Check sheet for the modelled part. Datum: model origin and axes. Units: mm. Face numbers are marked on the shaded views. A direction names the side the tool comes from. Round coordinates to 2 decimals unless told otherwise and drop trailing zeros. Write each loop counter-clockwise with the first axis right and the second up, starting at its lowest first coordinate (ties: lowest second). Pieces come first, ordered by that corner, then holes.
Item 1: Cross-section at C-C on z = 14.25. Enter the section's corners in (x, y) (3 decimals).
Item 2: Cross-section at B-B on y = 38.1. Enter the section's corners in (x, z) (3 decimals).
Item 3: Release check for a two-part mould opening along Z. For the marked faces 1, 2, 3 and 4 record: +Z half, -Z half, draft (parallel to the pull), parting line (faces both ways), or undercut.
Item 4: Go/stop test with a flat-tipped pin: pin 1 Ø5 at (x, y) = (38.1, 38.1) entering from +Z. Record where the tip stops, or that it passes through.
Item 5: Cross-section at A-A on x = 25.4. Enter the section's corners in (y, z) (3 decimals).
Item 6: Tool access check on the marked faces 5 and 6. Record the directions out of +Z, -Z, +X, -X, +Y, -Y that give a thin tool (end or side, any length) a straight path to the whole face; none if there is none.
Item 7: Cross-section at D-D on x = 12.7. Count the separate pieces of the cut face and the enclosed holes in it, plus the area to 3 significant figures.
Item 8: Material ranges on line 1 (X direction, y = 38.1, z = 23.5) (3 decimals); line 2 (X direction, y = 46, z = 17.75) (3 decimals); line 3 (Z direction, x = 47.5, y = 93.5) (3 decimals), recorded low to high.
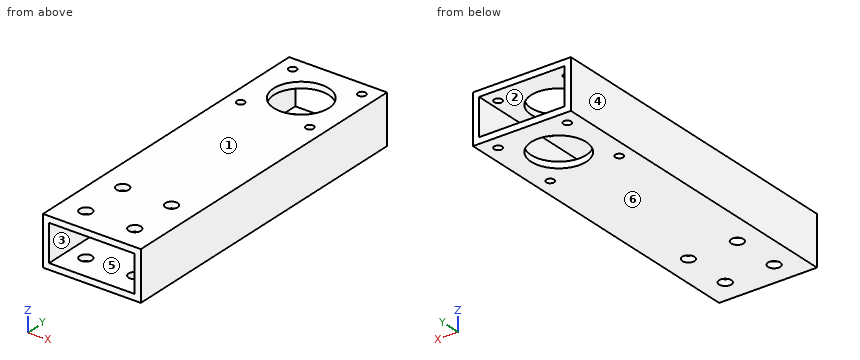
Autodesk Inventor part; units mm, degrees
ref_plane "YZ Plane" through (0, 0, 0) normal (1, 0, 0) x (0, 1, 0)
ref_plane "XZ Plane" through (0, 0, 0) normal (0, 1, 0) x (-1, 0, 0)
ref_plane "XY Plane" through (0, 0, 0) normal (0, 0, 1) x (1, 0, 0)
sketch "Sketch1" plane through (0, 0, 0) normal (0, 0, 1) x (1, 0, 0)
  line L0 (0, 0) -> (50.8, 0)
  line L1 (50.8, 0) -> (50.8, 169.8752)
  line L2 (50.8, 169.8752) -> (0, 169.8752)
  line L3 (0, 169.8752) -> (0, 0)
  line L4 (25.4, 169.8752) -> (25.4, 144.4752)
  line L5 (25.4, 169.8752) -> (50.8, 169.8752) construction
  circle A0 centre (25.4, 144.4752) radius 14.2875
  line L6 (25.4, 144.4752) -> (43.3605, 162.4357)
  line L7 (25.4, 144.4752) -> (50.8, 144.4752) construction
  line L8 (7.4395, 126.5147) -> (43.3605, 126.5147)
  line L9 (43.3605, 162.4357) -> (7.4395, 162.4357)
  line L10 (7.4395, 162.4357) -> (7.4395, 126.5147)
  circle A1 centre (7.4395, 162.4357) radius 2.032
  circle A2 centre (7.4395, 126.5147) radius 2.032
  circle A3 centre (43.3605, 162.4357) radius 2.032
  circle A4 centre (43.3605, 126.5147) radius 2.032
  line L11 (0, 0) -> (50.8, 0)
  line L12 (50.8, 0) -> (50.8, 38.1)
  line L13 (0, 38.1) -> (0, 0)
  line L14 (25.4, 38.1) -> (12.7, 38.1)
  line L15 (25.4, 38.1) -> (38.1, 38.1) construction
  line L16 (12.7, 38.1) -> (38.1, 38.1)
  circle A5 centre (12.7, 38.1) radius 3.175
  circle A6 centre (38.1, 38.1) radius 3.175
  dimension "d0" = 50.8
  dimension "d1" = 169.8752
  dimension "d2" = 25.4
  dimension "d3" = 90
  dimension "d4" = 28.575
  dimension "d5" = 25.4
  dimension "d6" = 45
  dimension "d7" = 50.8
  dimension "d9" = 4.064
  dimension "d10" = 4.064
  dimension "d11" = 4.064
  dimension "d12" = 4.064
  dimension "d13" = 50.8
  dimension "d14" = 38.1
  dimension "d15" = 12.7
  dimension "d16" = 180
  dimension "d17" = 25.4
  dimension "d18" = 0
  dimension "d19" = 6.35
  dimension "d20" = 6.35
extrude "Extrusion1" add sketch "Sketch1" along normal blind 25.4 contours L9 A3 L6 A0 L4 | L3 L2 L1 L0
sketch "Sketch2" plane through (0, 169.8752, 0) normal (0, 1, 0) x (1, 0, 0)
  line L0 (0, 0) -> (3.175, 0)
  line L1 (3.175, 0) -> (3.175, -3.175)
  line L2 (3.175, -3.175) -> (0, -3.175)
  line L3 (0, -3.175) -> (0, 0)
  line L4 (3.175, -3.175) -> (47.625, -3.175)
  line L5 (47.625, -3.175) -> (47.625, -22.225)
  line L6 (47.625, -22.225) -> (3.175, -22.225)
  line L7 (3.175, -22.225) -> (3.175, -3.175)
  dimension "d23" = 3.175
  dimension "d24" = 3.175
  dimension "d25" = 44.45
  dimension "d26" = 19.05
extrude "Extrusion2" cut sketch "Sketch2" against normal blind 254 contours L4 L5 L6 L7
sketch "Sketch3" plane through (0, 0, 25.4) normal (0, 0, 1) x (1, 0, 0)
  circle A0 centre (12.7, 38.1) radius 3.175
  line L0 (12.7, 38.1) -> (38.1, 38.1)
  line L1 (38.1, 38.1) -> (38.1, 12.7)
  line L2 (38.1, 12.7) -> (12.7, 12.7)
  line L3 (12.7, 12.7) -> (12.7, 38.1)
  circle A1 centre (12.7, 12.7) radius 3.175
  circle A2 centre (38.1, 12.7) radius 3.175
  dimension "d29" = 25.4
  dimension "d30" = 25.4
  dimension "d31" = 6.35
  dimension "d32" = 6.35
extrude "Extrusion3" cut sketch "Sketch3" against normal blind 25.4 contours A1 L2 L3 | L3 L2 A1 | A2 L2 L1 | L1 L2 A2
properties part number "Z-Bar"
Response values:
1. outline: (0, 0) - (3.175, 0) - (3.175, 169.875) - (0, 169.875) - close; (47.625, 0) - (50.8, 0) - (50.8, 169.875) - (47.625, 169.875) - close
2. outline: (0, 0) - (9.525, 0) - (9.525, 3.175) - (3.175, 3.175) - (3.175, 22.225) - (9.525, 22.225) - (9.525, 25.4) - (0, 25.4) - close; (15.875, 0) - (34.925, 0) - (34.925, 3.175) - (15.875, 3.175) - close; (15.875, 22.225) - (34.925, 22.225) - (34.925, 25.4) - (15.875, 25.4) - close; (41.275, 0) - (50.8, 0) - (50.8, 25.4) - (41.275, 25.4) - (41.275, 22.225) - (47.625, 22.225) - (47.625, 3.175) - (41.275, 3.175) - close
3. face 1: +Z half
3. face 2: undercut
3. face 3: undercut
3. face 4: draft
4. pin 1: passes through
5. outline: (0, 0) - (130.188, 0) - (130.188, 3.175) - (0, 3.175) - close; (0, 22.225) - (130.188, 22.225) - (130.188, 25.4) - (0, 25.4) - close; (158.763, 0) - (169.875, 0) - (169.875, 3.175) - (158.763, 3.175) - close; (158.763, 22.225) - (169.875, 22.225) - (169.875, 25.4) - (158.763, 25.4) - close
6. face 5: +Y, -Y
6. face 6: -Z, +X, -X, +Y, -Y
7. separate pieces: 8
7. enclosed holes: 0
7. area: 915 mm2
8. line 1: x = 0 to 9.525, 15.875 to 34.925, 41.275 to 50.8
8. line 2: x = 0 to 3.175, 47.625 to 50.8
8. line 3: z = 0 to 3.175, 22.225 to 25.4
